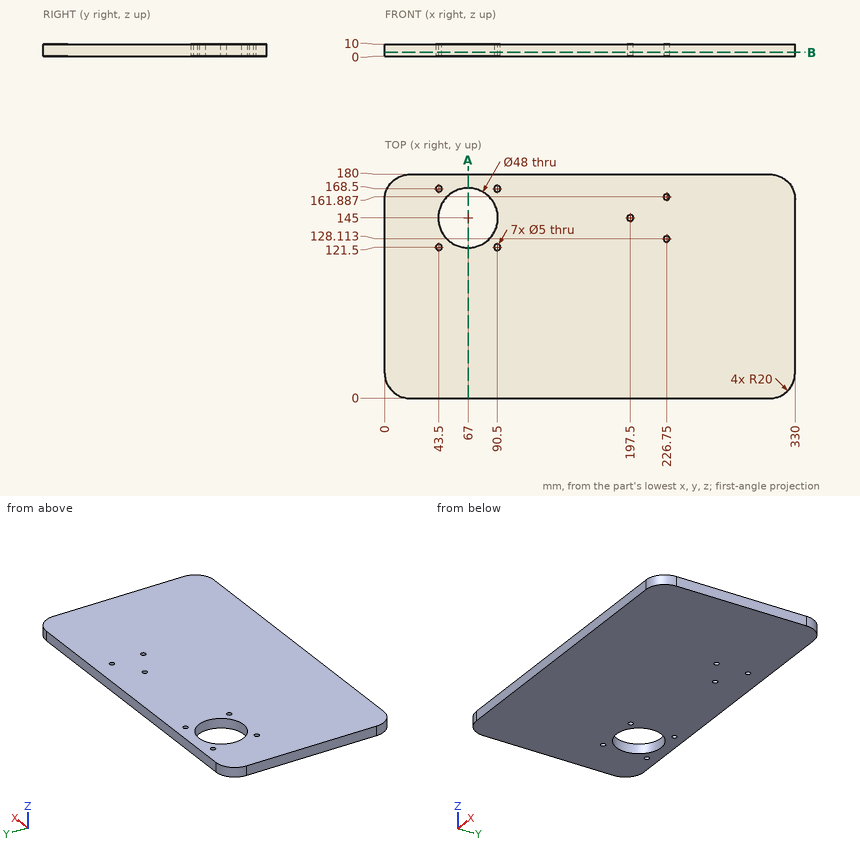
The drawing under review shows one solid part. Ordinate dimensions are in mm from its lowest x, y, z. Coordinates: 2 decimals unless noted, no trailing zeros. Loops run counter-clockwise (first coordinate to the right, second up) from the corner with the lowest first, then second, coordinate; pieces in that order, holes last.
Item 1: Add section A-A (x = 67). Write out the cut boundary in (y, z).
Completed:
outline: (0, 0) - (121, 0) - (121, 10) - (0, 10) - close; (169, 0) - (180, 0) - (180, 10) - (169, 10) - close
Item 2: Clearance check with a flat-ended pin moving along its axis: pin 1 (4 mm diameter, centred on x = 226.75, y = 128.11, fed in from +Z). State where the tip first meets the part, or that it passes through.
Completed:
pin 1: passes through
Item 3: Add section B-B (z = 3.25). Give the number of separate pieces and of enclosed holes in the cut face, and give its area (3 significant figures).
Completed:
separate pieces: 1
enclosed holes: 8
area: 57,100 mm2
Item 4: Wall thickness on L1, parallel to Y at x = 226.75, z = 4.75; L2, parallel to X at y = 144, z = 8.5; L3, parallel to Y at x = 92.5, z = 5.5: over which ranges is each line inside the solid? List them lowest first.
Completed:
L1: y = 0 to 125.61, 130.61 to 159.39, 164.39 to 180
L2: x = 0 to 43.02, 90.98 to 195.21, 199.79 to 330
L3: y = 0 to 120, 123 to 167, 170 to 180
